Source: CAD feature listing. Evaluate the final solid. Frame: model axes, mm. Round coordinates to 2 decimals unless told otherwise and drop trailing zeros. Write each loop counter-clockwise with the first axis right and the second up, starting at its lowest first coordinate (ties: lowest second). Pieces come first, ordered by that corner, then holes.
from build123d import *

# Parameters (mm, degrees)
SKETCH1_W             = 150
SKETCH1_H             = 70
SKETCH1_R             = 1.725
SKETCH1_R_2           = 1.13
BOSS_EXTRUDE1_DEPTH   = 4.7752
F_4_40_TAPPED_HOLE1_D = 2.2606


with BuildPart() as part:
    # Sketch1 → Boss-Extrude1 (new body)
    with BuildSketch(Plane.XY):
        with Locations((75, -35)):
            Rectangle(SKETCH1_W, SKETCH1_H)
        with Locations((7.5, -7.5)):
            Circle(SKETCH1_R, mode=Mode.SUBTRACT)
        with Locations((142.5, -7.5)):
            Circle(SKETCH1_R, mode=Mode.SUBTRACT)
        with Locations((142.5, -62.5)):
            Circle(SKETCH1_R, mode=Mode.SUBTRACT)
        with Locations((7.5, -62.5)):
            Circle(SKETCH1_R, mode=Mode.SUBTRACT)
        with Locations((7.5, -13.5)):
            Circle(SKETCH1_R_2, mode=Mode.SUBTRACT)
        with Locations((142.5, -13.5)):
            Circle(SKETCH1_R_2, mode=Mode.SUBTRACT)
        with Locations((142.5, -56.5)):
            Circle(SKETCH1_R_2, mode=Mode.SUBTRACT)
        with Locations((7.5, -56.5)):
            Circle(SKETCH1_R_2, mode=Mode.SUBTRACT)
        with Locations((40, -10)):
            Circle(SKETCH1_R, mode=Mode.SUBTRACT)
        with Locations((40, -60)):
            Circle(SKETCH1_R, mode=Mode.SUBTRACT)
        with Locations((110, -10)):
            Circle(SKETCH1_R, mode=Mode.SUBTRACT)
        with Locations((110, -60)):
            Circle(SKETCH1_R, mode=Mode.SUBTRACT)
    extrude(amount=BOSS_EXTRUDE1_DEPTH)

    # #4-40 Tapped Hole1 (through all)
    with Locations(Plane(origin=(7.5, -13.5, 4.7752), x_dir=(1, 0, 0), z_dir=(0, 0, 1))):
        with Locations((0, 0), (0, -43), (135, -43), (135, 0)):
            Hole(F_4_40_TAPPED_HOLE1_D / 2)


solid = part.part
1) Pull-direction query (X, two-part tool) for faces 1 (the face through (39.78, -8.29, 2.35)), 2 (the face through (74, -35, 4.775)), 3 (the face through (39.78, -58.29, 2.35)), 4 (the face through (150, -35, 2)); classes: released by +X, released by -X, zero draft, split by the parting line, or undercut.
Taken from the geometry:
face 1: undercut
face 2: zero draft
face 3: undercut
face 4: released by +X
2) Section query A-A on x = 110. Return the cut outline in (y, z) (3 decimals), then the cut area to 3 significant figures.
Taken from the geometry:
outline: (-70, 0) - (-61.725, 0) - (-61.725, 4.775) - (-70, 4.775) - close; (-58.275, 0) - (-11.725, 0) - (-11.725, 4.775) - (-58.275, 4.775) - close; (-8.275, 0) - (0, 0) - (0, 4.775) - (-8.275, 4.775) - close
area: 301 mm2
3) Material intervals for line 1 (Y direction, x = 7.5, z = 3.3) (3 decimals); line 2 (Y direction, x = 40, z = 2.2) (3 decimals); line 3 (Y direction, x = 41.5, z = 4.3), sorted ascending.
Taken from the geometry:
line 1: y = -70 to -64.225, -60.775 to -57.63, -55.37 to -14.63, -12.37 to -9.225, -5.775 to 0
line 2: y = -70 to -61.725, -58.275 to -11.725, -8.275 to 0
line 3: y = -70 to -60.85, -59.15 to -10.85, -9.15 to 0
